```python
from build123d import *

# Parameters (mm, degrees)
SKETCH1_R           = 30
BOSS_EXTRUDE1_DEPTH = 3
SKETCH2_R           = 10
BOSS_EXTRUDE2_DEPTH = 10
SKETCH3_R           = 5
BOSS_EXTRUDE3_DEPTH = 10
SKETCH6_R           = 2
CUT_EXTRUDE1_DEPTH  = 49.259714048
CUT_EXTRUDE2_REACH  = 50.26
SKETCH7_R           = 4.25
SKETCH7_R_2         = 2.5
SKETCH8_R           = 1.5
CUT_EXTRUDE3_DEPTH  = 15
FILLET1_R           = 1
CHAMFER1_SIZE       = 1
CHAMFER2_SIZE       = 1


with BuildPart() as part:
    # Sketch1 → Boss-Extrude1 (new body)
    with BuildSketch(Plane(origin=(0, 0, 0), x_dir=(0, 0, -1), z_dir=(1, 0, 0))):
        Circle(SKETCH1_R)
    extrude(amount=-BOSS_EXTRUDE1_DEPTH)

    # Sketch2 → Boss-Extrude2 (add)
    with BuildSketch(Plane(origin=(0, 0, 0), x_dir=(0, 0, -1), z_dir=(1, 0, 0))):
        Circle(SKETCH2_R)
    extrude(amount=BOSS_EXTRUDE2_DEPTH)

    # Sketch3 → Boss-Extrude3 (add)
    with BuildSketch(Plane(origin=(10, 0, 0), x_dir=(0, 0, -1), z_dir=(1, 0, 0))):
        Circle(SKETCH3_R)
    extrude(amount=BOSS_EXTRUDE3_DEPTH)

    # Sketch4 → Cut-Revolve1 (revolve, cut)
    with BuildSketch(Plane.XY, mode=Mode.PRIVATE) as cut_revolve1_sk:
        Polygon((10, 5), (0, 10), (10, 10), align=None)
    revolve(cut_revolve1_sk.sketch.rotate(Axis((0, 0, 0), (1, 0, 0)), 90), axis=Axis((0, 0, 0), (1, 0, 0)), mode=Mode.SUBTRACT)

    # Sketch6 → Cut-Extrude1 (cut, through all)
    with BuildSketch(Plane(origin=(20, 0, 0), x_dir=(0, 0, -1), z_dir=(1, 0, 0))):
        Circle(SKETCH6_R)
    extrude(amount=-CUT_EXTRUDE1_DEPTH, mode=Mode.SUBTRACT)

    # Sketch7 → Cut-Extrude2 (cut, up to next)
    with BuildSketch(Plane.ZY.offset(3), mode=Mode.PRIVATE) as cut_extrude2_sk1:
        with Locations((-11.875, 20.56810334)):
            Circle(SKETCH7_R)
    cut_extrude2_tool1 = extrude(cut_extrude2_sk1.sketch, amount=-CUT_EXTRUDE2_REACH, mode=Mode.PRIVATE) & part.part
    # Sketch7 → Cut-Extrude2 (cut, up to next)
    with BuildSketch(Plane.ZY.offset(3), mode=Mode.PRIVATE) as cut_extrude2_sk2:
        with Locations((23.75, 0)):
            Circle(SKETCH7_R)
    cut_extrude2_tool2 = extrude(cut_extrude2_sk2.sketch, amount=-CUT_EXTRUDE2_REACH, mode=Mode.PRIVATE) & part.part
    # Sketch7 → Cut-Extrude2 (cut, up to next)
    with BuildSketch(Plane.ZY.offset(3), mode=Mode.PRIVATE) as cut_extrude2_sk3:
        with Locations((-11.875, -20.56810334)):
            Circle(SKETCH7_R)
    cut_extrude2_tool3 = extrude(cut_extrude2_sk3.sketch, amount=-CUT_EXTRUDE2_REACH, mode=Mode.PRIVATE) & part.part
    # Sketch7 → Cut-Extrude2 (cut, up to next)
    with BuildSketch(Plane.ZY.offset(3), mode=Mode.PRIVATE) as cut_extrude2_sk4:
        with Locations((11.875, 20.56810334)):
            Circle(SKETCH7_R_2)
    cut_extrude2_tool4 = extrude(cut_extrude2_sk4.sketch, amount=-CUT_EXTRUDE2_REACH, mode=Mode.PRIVATE) & part.part
    # Sketch7 → Cut-Extrude2 (cut, up to next)
    with BuildSketch(Plane.ZY.offset(3), mode=Mode.PRIVATE) as cut_extrude2_sk5:
        with Locations((11.875, -20.56810334)):
            Circle(SKETCH7_R_2)
    cut_extrude2_tool5 = extrude(cut_extrude2_sk5.sketch, amount=-CUT_EXTRUDE2_REACH, mode=Mode.PRIVATE) & part.part
    # Sketch7 → Cut-Extrude2 (cut, up to next)
    with BuildSketch(Plane.ZY.offset(3), mode=Mode.PRIVATE) as cut_extrude2_sk6:
        with Locations((-23.75, 0)):
            Circle(SKETCH7_R_2)
    cut_extrude2_tool6 = extrude(cut_extrude2_sk6.sketch, amount=-CUT_EXTRUDE2_REACH, mode=Mode.PRIVATE) & part.part
    add(cut_extrude2_tool1.solids().sort_by_distance((-3, 20.568103, -11.875))[0], mode=Mode.SUBTRACT)
    add(cut_extrude2_tool2.solids().sort_by_distance((-3, 0, 23.75))[0], mode=Mode.SUBTRACT)
    add(cut_extrude2_tool3.solids().sort_by_distance((-3, -20.568103, -11.875))[0], mode=Mode.SUBTRACT)
    add(cut_extrude2_tool4.solids().sort_by_distance((-3, 20.568103, 11.875))[0], mode=Mode.SUBTRACT)
    add(cut_extrude2_tool5.solids().sort_by_distance((-3, -20.568103, 11.875))[0], mode=Mode.SUBTRACT)
    add(cut_extrude2_tool6.solids().sort_by_distance((-3, 0, -23.75))[0], mode=Mode.SUBTRACT)

    # Sketch8 → Cut-Extrude3 (cut)
    with BuildSketch(Plane(origin=(0, 0, 0), x_dir=(1, 0, 0), z_dir=(0, 1, 0))):
        with Locations(Location((15, 0, 0), (0, 0, 90))):
            Circle(SKETCH8_R)
    extrude(amount=CUT_EXTRUDE3_DEPTH, mode=Mode.SUBTRACT)

    # Fillet1
    fillet1_edges = [part.edges().sort_by_distance(p)[0] for p in [
        (20, 0, 5),
    ]]
    fillet(fillet1_edges, radius=FILLET1_R)

    # Chamfer1
    chamfer1_edges = [part.edges().sort_by_distance(p)[0] for p in [
        (-3, 0, 30),
    ]]
    chamfer(chamfer1_edges, length=CHAMFER1_SIZE)

    # Chamfer2
    chamfer2_edges = [part.edges().sort_by_distance(p)[0] for p in [
        (-3, 0, 2),
    ]]
    chamfer(chamfer2_edges, length=CHAMFER2_SIZE)


solid = part.part
```
Source: CAD feature listing. Evaluate the final solid. Frame: model axes, mm. A direction names the side the tool comes from. Give positions to 0.01 mm unless a question says otherwise; leave off trailing zeros. Loops run counter-clockwise (first coordinate to the right, second up) from the corner with the lowest first, then second, coordinate; pieces in that order, holes last. Notation, with made-up numbers: M 70,78.25 L 84,78.25 A15 cw 84,100.25 Z; hole C 14.5,52 d1. An arc over 180 degrees is marked long. Put each result on its own line as item: value.
Q1. Reachability of faces 4 (the cylindrical face through (14.55, 3.14, -1.43)), 5 (the cylindrical face through (-1.521, 23.047, 11.55)), 6 (the flat face through (0, 0, -13)) from +Z, -Z, +X, -X, +Y, -Y: full face, straight path, thin tool, end or side. Return the list, or none.
Response values:
face 4: +Y
face 5: +X, -X
face 6: +X
Q2. Section D-D (x = 15). Return the cut outline in (y, z), and give its area (3 significant figures).
Response values:
outline: M 1.32,-1.5 A2 cw long 1.32,1.5 L 4.77,1.5 A5 ccw long 4.77,-1.5 Z
area: 56.6 mm²
Q3. Line query: probe 1 along Y at (x, z) = (-2.05, -23.75); probe 2 along Z at (x, y) = (9.75, -0.5); probe 3 along Z at (x, y) = (-1.5, -3.5). Output: solid intervals per line, ascending. Write a range as [from, to].
Response values:
probe 1: y = [-18.25, -2.5], [2.5, 18.25]
probe 2: z = [-5.1, -1.94], [1.94, 5.1]
probe 3: z = [-29.8, 21.34], [26.16, 29.8]
Q4. Mould query, pull axis Z, two halves, no side actions, for faces 1 (the cylindrical face through (14.44, -4.88, 1.08)), 2 (the cylindrical face through (-1.521, -24.717, -12.796)), 3 (the flat face through (-3, 0, -6)). Classes: released by +Z, released by -Z, zero draft, split by the parting line, or undercut.
Response values:
face 1: split by the parting line
face 2: undercut
face 3: zero draft
Q5. Section C-C (x = 1.25). Return the cut outline in (y, z) (3 decimals).
Response values:
outline: C 0,0 d18.75; hole C 0,0 d4
Q6. Section A-A (y = 0). Return the cut outline in (x, z).
Response values:
outline: M -3,-29 L -2,-30 L 0,-30 L 0,-26.25 L -3,-26.25 Z; M -3,-21.25 L 0,-21.25 L 0,-10 L 10,-5 L 19,-5 A1 ccw 20,-4 L 20,-2 L -2,-2 L -3,-3 Z; M -3,3 L -2,2 L 20,2 L 20,4 A1 ccw 19,5 L 10,5 L 0,10 L 0,19.5 L -3,19.5 Z; M -3,28 L 0,28 L 0,30 L -2,30 L -3,29 Z
Q7. Section B-B (z = 0). Return the cut outline in (x, y), and give its area (3 significant figures).
Response values:
outline: M -3,-29 L -2,-30 L 0,-30 L 0,-10 L 10,-5 L 19,-5 A1 ccw 20,-4 L 20,-2 L -2,-2 L -3,-3 Z; M -3,3 L -2,2 L 13.5,2 L 13.5,5 L 10,5 L 0,10 L 0,30 L -2,30 L -3,29 Z; M 16.5,2 L 20,2 L 20,4 A1 ccw 19,5 L 16.5,5 Z
area: 327 mm²
Q8. Pin query (flat end, axial travel): P1, Ø10, axis at x = 7, y = -0.5, coming from the -Z side; P2, Ø2, axis at y = 16.5, z = -14, coming from the +X side; P3, Ø11, axis at y = -20.57, z = -11.88, coming from the -X side; P4, Ø4.5, axis at y = 20.57, z = 11.88, coming from the -X side. Return the tip coordinate at first contact, or that it passes through.
Response values:
P1: stops at z = -8.99
P2: stops at x = 0
P3: stops at x = -3
P4: passes through
